Source: CAD feature listing. Evaluate the final solid. Frame: model axes, mm. Give positions to 0.01 mm unless a question says otherwise; leave off trailing zeros. Order: outer loops, then holes, each group sorted by start corner. A loop starts at its lowest first (then second) coordinate and runs counter-clockwise, first axis right, second up.
```python
from build123d import *

# Parameters (mm, degrees)
SKETCH1_R           = 2.5
BOSS_EXTRUDE1_DEPTH = 6
FILLET1_R           = 3


with BuildPart() as part:
    # Sketch1 → Boss-Extrude1 (new body)
    with BuildSketch(Plane.XY):
        with BuildLine():
            Line((-21, 11.584180911), (21, 11.584180911))
            ThreePointArc((21, 11.584180911), (23.828427125, 10.412608036), (25, 7.584180911))
            Line((25, 7.584180911), (25, -4.415819089))
            ThreePointArc((25, -4.415819089), (23.828427125, -7.244246214), (21, -8.415819089))
            Line((21, -8.415819089), (-21, -8.415819089))
            ThreePointArc((-21, -8.415819089), (-23.828427125, -7.244246214), (-25, -4.415819089))
            Line((-25, -4.415819089), (-25, 7.584180911))
            ThreePointArc((-25, 7.584180911), (-23.828427125, 10.412608036), (-21, 11.584180911))
        make_face()
        with Locations((0, 1.584180911)):
            Circle(SKETCH1_R, mode=Mode.SUBTRACT)
    extrude(amount=BOSS_EXTRUDE1_DEPTH)

    # Fillet1
    fillet1_edges = [part.edges().sort_by_distance(p)[0] for p in [
        (-25, 1.584180911, 0),
        (-23.828427125, 10.412608036, 0),
        (0, 11.584180911, 0),
        (23.828427125, 10.412608036, 0),
        (25, 1.584180911, 0),
        (23.828427125, -7.244246214, 0),
        (0, -8.415819089, 0),
        (-23.828427125, -7.244246214, 0),
    ]]
    fillet(fillet1_edges, radius=FILLET1_R)


solid = part.part
```
1) Section query C-C, the plane z = 4.4. Return the cut outline in (x, y), and give its area (3 significant figures).
Report:
outline: (-25, -4.42) arc R4 ccw to (-21, -8.42) - (21, -8.42) arc R4 ccw to (25, -4.42) - (25, 7.58) arc R4 ccw to (21, 11.58) - (-21, 11.58) arc R4 ccw to (-25, 7.58) - close; hole circle Ø5 at (0, 1.58)
area: 967 mm2
2) Section query B-B, the plane y = 0.75. Return the cut outline in (x, z).
Report:
outline: (-25, 3) arc R3 ccw to (-22, 0) - (-2.36, 0) - (-2.36, 6) - (-25, 6) - close; (2.36, 0) - (22, 0) arc R3 ccw to (25, 3) - (25, 6) - (2.36, 6) - close
3) Section query A-A, the plane x = 0. Return the cut outline in (y, z).
Report:
outline: (-8.42, 3) arc R3 ccw to (-5.42, 0) - (-0.92, 0) - (-0.92, 6) - (-8.42, 6) - close; (4.08, 0) - (8.58, 0) arc R3 ccw to (11.58, 3) - (11.58, 6) - (4.08, 6) - close
4) Draft query along X for faces 1 (the cylindrical face through (-0.542, -0.856, 2.958)), 2 (the cylindrical face through (0.294, 10.729, 0.902)), 3 (the cylindrical face through (23.86, -7.21, 4.48)), 4 (the cylindrical face through (-23.797, -7.275, 4.479)). Return one class per face: +X half, -X half, draft (parallel to the pull), parting line (faces both ways), or undercut.
Report:
face 1: undercut
face 2: draft
face 3: +X half
face 4: -X half
5) Section query D-D, the plane x = 20.5. Return the cut outline in (y, z).
Report:
outline: (-8.42, 3) arc R3 ccw to (-5.42, 0) - (8.58, 0) arc R3 ccw to (11.58, 3) - (11.58, 6) - (-8.42, 6) - close
6) Material intervals for L1, parallel to Y at x = 0, z = 3; L2, parallel to Z at x = -17.5, y = -5.5; L3, parallel to Y at x = 0, z = 1.3, sorted ascending.
Report:
L1: y = -8.42 to -0.92, 4.08 to 11.58
L2: z = 0 to 6
L3: y = -7.89 to -0.92, 4.08 to 11.06
